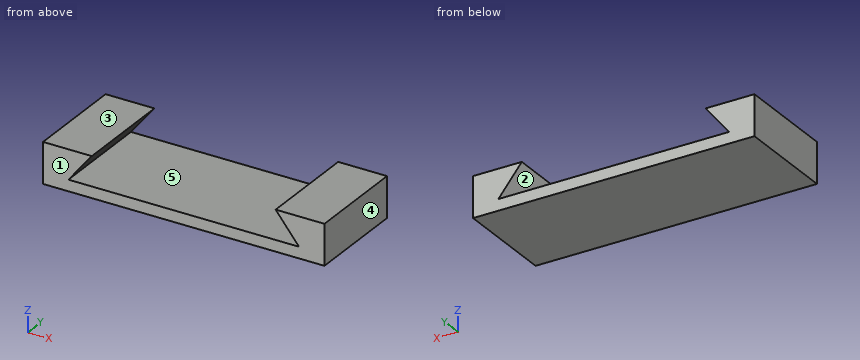
Autodesk Fusion 360 part; units mm, degrees
ref_plane "工作平面1" through (0, 0, 0) normal (0, 0, 1) x (1, 0, 0)
sketch "草图1" plane through (0, 0, 0) normal (0, 0, 1) x (1, 0, 0)
  line L0 (-25, -9) -> (25, -9)
  line L1 (25, -9) -> (25, 9)
  line L2 (25, 9) -> (-25, 9)
  line L3 (-25, 9) -> (-25, -9)
extrude "Coupon base" add sketch "草图1" along normal blind 2
ref_plane "工作平面2" through (0, 0, 2) normal (0, 0, 1) x (1, 0, 0)
sketch "草图2" plane through (0, 0, 2) normal (0, 0, 1) x (1, 0, 0)
  line L0 (-25, -9) -> (-20.49, -9)
  line L1 (-20.49, -9) -> (-20.49, 9)
  line L2 (-20.49, 9) -> (-25, 9)
  line L3 (-25, 9) -> (-25, -9)
ref_plane "工作平面3" through (0, 0, 7.2) normal (0, 0, 1) x (1, 0, 0)
sketch "草图3" plane through (0, 0, 7.2) normal (0, 0, 1) x (1, 0, 0)
  line L0 (-25, -9) -> (-16.33, -9)
  line L1 (-16.33, -9) -> (-16.33, 9)
  line L2 (-16.33, 9) -> (-25, 9)
  line L3 (-25, 9) -> (-25, -9)
loft "Coupon dovetail rail" add profiles "草图2", "草图3" section 1 section 2
ref_plane "工作平面4" through (0, 0, 2) normal (0, 0, 1) x (1, 0, 0)
sketch "草图4" plane through (0, 0, 2) normal (0, 0, 1) x (1, 0, 0)
  line L0 (20.49, -9) -> (25, -9)
  line L1 (25, -9) -> (25, 9)
  line L2 (25, 9) -> (20.49, 9)
  line L3 (20.49, 9) -> (20.49, -9)
ref_plane "工作平面5" through (0, 0, 7.2) normal (0, 0, 1) x (1, 0, 0)
sketch "草图5" plane through (0, 0, 7.2) normal (0, 0, 1) x (1, 0, 0)
  line L0 (16.33, -9) -> (25, -9)
  line L1 (25, -9) -> (25, 9)
  line L2 (25, 9) -> (16.33, 9)
  line L3 (16.33, 9) -> (16.33, -9)
loft "Coupon dovetail rail (1)" add profiles "草图4", "草图5" section 1 section 2
Here's how the part is built. I have some questions about the finished solid (model axes, mm). Face numbers are marked on the shaded views. A direction names the side the tool comes from. Give positions to 0.01 mm unless a question says otherwise; leave off trailing zeros. Write each loop counter-clockwise with the first axis right and the second up, starting at its lowest first coordinate (ties: lowest second). Pieces come first, ordered by that corner, then holes. Notation, with made-up numbers: M 14.5,67.25 L 57.5,67.25 A13 cw 57.5,90.25 Z; hole C 24.5,18 d10. An arc over 180 degrees is marked long. Put each result on its own line as item: value. Start each with the question number.
Item 1: On a 3-axis mill with a long thin cutter (end or side, diameter ignored), from which of +Z, -Z, +X, -X, +Y, -Y can I reach the whole of each face in a straight line? I mean the marked faces 4 and 5. Say none if no direction works.
Item 2: Thinking about a two-plate mould opening in Z: for the marked faces 1, 2 and 3, which applies, +Z half, -Z half, draft (parallel to the pull), parting line (faces both ways), or undercut?
Item 3: Will this pin go through, and if not, where does the flat tip stop? pin 1 (1.5 mm diameter, centred on x = 10.5, y = -5.5, fed in from +Z).
Item 4: If we section it at D-D, the plane x = 6: Write out the boundary of the cut face in (y, z).
Item 5: I need wall thicknesses on L1, parallel to Z at x = 6.5, y = -1.5; L2, parallel to X at y = -3, z = 2.5; L3, parallel to X at y = -7, z = 2.25. Which ranges of each line are inside material? Lowest first, please. Write a range as from..to.
Item 6: If we section it at A-A, the plane z = 4.25: Write out the boundary of the cut face in (x, y), then the cut area to 3 significant figures.
Item 7: If we section it at B-B, the plane x = 20: Write out the boundary of the cut face in (y, z), then the cut area to 3 significant figures.
Item 8: If we section it at C-C, the plane y = -0.5: Write out the boundary of the cut face in (x, z), then the cut area to 3 significant figures.
Values:
1. face 4: +Z, -Z, +X, +Y, -Y
1. face 5: +Y, -Y
2. face 1: draft
2. face 2: undercut
2. face 3: +Z half
3. pin 1: z = 2
4. outline: M -9,0 L 9,0 L 9,2 L -9,2 Z
5. L1: 0..2
5. L2: -25..-20.09, 20.09..25
5. L3: -25..-20.29, 20.29..25
6. outline: M -25,-9 L -18.69,-9 L -18.69,9 L -25,9 Z; M 18.69,-9 L 25,-9 L 25,9 L 18.69,9 Z
6. area: 227 mm²
7. outline: M -9,0 L 9,0 L 9,2 L -9,2 Z; M -9,2.61 L 9,2.61 L 9,7.2 L -9,7.2 Z
7. area: 119 mm²
8. outline: M -25,0 L 25,0 L 25,7.2 L 16.33,7.2 L 20.49,2 L -20.49,2 L -16.33,7.2 L -25,7.2 Z
8. area: 169 mm²
